```python
from build123d import *

# Parameters (mm, degrees)
F3_DEPTH = 25
F4_DEPTH = 25


with BuildPart() as f1:
    # F0 (on Front) → F1 (revolve)
    with BuildSketch(Plane.XZ):
        Polygon((0, 31.622777), (0, 35.721142), (-18, 0), (-18, -28), (0, -28), (0, -25), (-15, -25), (-15, 0), align=None)
    revolve(axis=Axis((0, 0, 3.311388), (0, 0, -1)))

    # F2 (on Front) → F3 (cut)
    with BuildSketch(Plane.XZ):
        Polygon((0, 33.6782), (-14.015529, 0), (14.151254, 0), align=None)
    extrude(amount=-F3_DEPTH, mode=Mode.SUBTRACT)

    # F2 (on Front) → F4 (cut)
    with BuildSketch(Plane.XZ):
        Polygon((0, 33.6782), (-14.015529, 0), (14.151254, 0), align=None)
    extrude(amount=F4_DEPTH, mode=Mode.SUBTRACT)


solid = f1.part
```
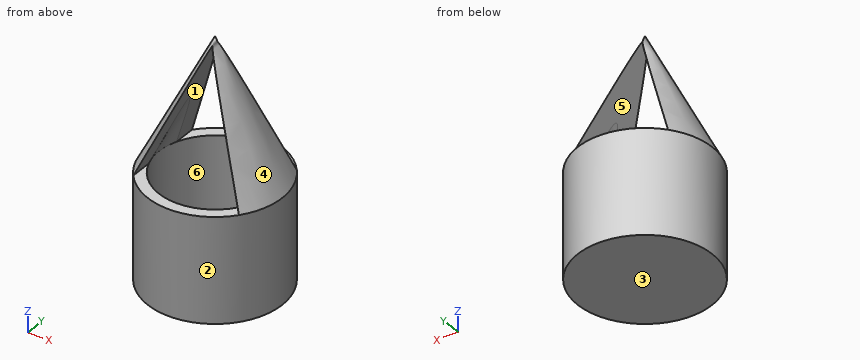
Could you check a few things on this model? Use its own coordinates, in mm. Face numbers are marked on the shaded views. A direction names the side the tool comes from. Give positions to 0.01 mm unless a question says otherwise; leave off trailing zeros. Order: outer loops, then holes, each group sorted by start corner. A loop starts at its lowest first (then second) coordinate and runs counter-clockwise, first axis right, second up.
Q1. Suppose I cut it at D-D, the plane y = -16. Write out the boundary of the cut face in (x, z).
Q2. We'd pull the mould along Z, two halves only. Please class the marked faces 1, 2 and 3: +Z half, -Z half, draft (parallel to the pull), parting line (faces both ways), or undercut.
Q3. Suppose I cut it at B-B, the plane z = -20. Write out the boundary of the cut face in (x, y).
Q4. If I drill on line 1 along Y through (x, z) = (0, -9.5); line 2 along Y through (x, z) = (12, -19.5), over which ranges is the centre line in solid material (lowest first)?
Q5. Suppose I cut it at A-A, the plane z = 13.5. Write out the boundary of the cut face in (x, y).
Q6. For the marked faces 4, 5 and 6, which set-ups out of +Z, -Z, +X, -X, +Y, -Y let a thin tool reach every point of the face, with its end or its side?
Q7. Suppose I cut it at C-C, the plane z = 3. Write out the boundary of the cut face in (x, y).
Q8. I'm going to push flat-ended pins straight in: P1, Ø1, axis at x = 12.5, y = -3, coming from the +Z side; P2, Ø6, axis at y = -14, z = -12, coming from the +X side; P3, Ø12, axis at y = 11, z = 21, coming from the +X side; P4, Ø2, axis at x = -5, z = 14.5, coming from the +Y side. Where does each tip first touch, or does it pass through?
Solution:
1. outline: (-8.25, -28) - (8.25, -28) - (8.25, 0) - (-8.25, 0) - close
2. face 1: undercut
2. face 2: draft
2. face 3: -Z half
3. outline: circle Ø36 at (0, 0); hole circle Ø30 at (0, 0)
4. line 1: y = -18 to -15, 15 to 18
4. line 2: y = -13.42 to -9, 9 to 13.42
5. outline: (-8.4, -7.41) - (-8.4, -1.84) arc R8.6 cw to (-8.4, 1.84) - (-8.4, 7.41) arc R11.2 ccw to start; (8.48, -7.31) arc R11.2 ccw to (8.48, 7.31) - (8.48, 1.42) arc R8.6 cw to (8.48, -1.42) - close
6. face 4: +Z
6. face 5: +Y, -Y
6. face 6: none
7. outline: (-12.77, -10.43) - (-12.77, -4.62) arc R13.58 cw to (-12.77, 4.62) - (-12.77, 10.43) arc R16.49 ccw to start; (12.89, -10.28) arc R16.49 ccw to (12.89, 10.28) - (12.89, 4.26) arc R13.58 cw to (12.89, -4.26) - close
8. P1: stops at z = 11.2
8. P2: stops at x = 14.25
8. P3: stops at x = 6.84
8. P4: passes through
